Build history of the part. All positions in model axes, mm. Round coordinates to 2 decimals unless told otherwise and drop trailing zeros. Loops run counter-clockwise (first coordinate to the right, second up) from the corner with the lowest first, then second, coordinate; pieces in that order, holes last.
from build123d import *

# Parameters (mm, degrees)
BOSS_EXTRUDE1_DEPTH   = 1.5875
F_2_CLEARANCE_HOLE1_D = 2.4384
FILLET1_R             = 3


with BuildPart() as part:
    # Sketch1 → Boss-Extrude1 (new body)
    with BuildSketch(Plane(origin=(0, 0, 0), x_dir=(0, 0, -1), z_dir=(1, 0, 0))):
        Polygon((0, 0), (174, 0), (174, 23.5), (135, 23.5), (135, 10), (0, 10), align=None)
    extrude(amount=BOSS_EXTRUDE1_DEPTH)

    # #2 Clearance Hole1 (through all)
    with Locations(Plane(origin=(1.5875, 0, 0), x_dir=(0, 0, -1), z_dir=(1, 0, 0))):
        with Locations((4, 5), (170, 5)):
            Hole(F_2_CLEARANCE_HOLE1_D / 2)

    # Fillet1
    fillet1_edges = [part.edges().sort_by_distance(p)[0] for p in [
        (0.79375, 10, -135),
        (0.79375, 23.5, -135),
        (0.79375, 23.5, -174),
    ]]
    fillet(fillet1_edges, radius=FILLET1_R)


solid = part.part
(1) Slice it at A-A on x = 1.25. List the corners of the cut face in (y, z), plus the area to 3 significant figures.
Responses:
outline: (0, -174) - (20.5, -174) arc R3 ccw to (23.5, -171) - (23.5, -138) arc R3 ccw to (20.5, -135) - (13, -135) arc R3 cw to (10, -132) - (10, 0) - (0, 0) - close; hole circle Ø2.44 at (5, -170); hole circle Ø2.44 at (5, -4)
area: 2,260 mm2
(2) Probe line 1 (Y direction, x = 1.2, z = -4); line 2 (Y direction, x = 0.8, z = -170); line 3 (Y direction, x = 1.2, z = -22.5). List the from-to ranges inside material, lowest first.
Responses:
line 1: y = 0 to 3.78, 6.22 to 10
line 2: y = 0 to 3.78, 6.22 to 23.5
line 3: y = 0 to 10
(3) Slice it at C-C on z = -69. List the corners of the cut face in (x, y), plus the area to 3 significant figures.
Responses:
outline: (0, 0) - (1.59, 0) - (1.59, 10) - (0, 10) - close
area: 15.9 mm2
(4) Slice it at B-B on y = 18. List the corners of the cut face in (x, z).
Responses:
outline: (0, -174) - (1.59, -174) - (1.59, -135) - (0, -135) - close
(5) Pin check, flat tips, straight feed: P1, Ø1.5, axis at y = 5, z = -170, coming from the +X side; P2, Ø0.5, axis at x = 0.5, z = -63, coming from the +Y side. Stop position of each tip, or through.
Responses:
P1: passes through
P2: stops at y = 10
